```python
from build123d import *

# Parameters (mm, degrees)
LUMEN_REACH         = 11.007
SKETCH5_R           = 1.125
SKETCH6_R           = 3.044910248
SKETCH6_R_2         = 1.125
MINCHANNEL_DEPTH    = 6
BARBCHANNELFILLET_R = 1


with BuildPart() as part:
    # Sketch4 → Barb (revolve)
    with BuildSketch(Plane.XY, mode=Mode.PRIVATE) as barb_sk:
        Polygon((-8.593939394, 0), (-8.593939394, 4.75), (-2.593939394, 3.044910248), (-2.593939394, 0), align=None)
    revolve(barb_sk.sketch.rotate(Axis((0, 0, 0), (-1, 0, 0)), 90), axis=Axis((0, 0, 0), (-1, 0, 0)))

    # Sketch5 → Lumen (cut, up to next)
    with BuildSketch(Plane(origin=(-2.593939394, 0, 0), x_dir=(0, 0, -1), z_dir=(1, 0, 0)), mode=Mode.PRIVATE) as lumen_sk1:
        Circle(SKETCH5_R)
    lumen_tool1 = extrude(lumen_sk1.sketch, amount=-LUMEN_REACH, mode=Mode.PRIVATE) & part.part
    add(lumen_tool1.solids().sort_by_distance((-2.593939, 0, 0))[0], mode=Mode.SUBTRACT)

    # Sketch6 → MinChannel (add)
    with BuildSketch(Plane.ZY.offset(8.593939394)):
        Circle(SKETCH6_R)
        with Locations(Location((0, 0, 0), (0, 0, 180))):
            Circle(SKETCH6_R_2, mode=Mode.SUBTRACT)
    extrude(amount=MINCHANNEL_DEPTH)

    # BarbChannelFillet
    barbchannelfillet_edges = [part.edges().sort_by_distance(p)[0] for p in [
        (-8.593939394, 0, -3.044910248),
    ]]
    fillet(barbchannelfillet_edges, radius=BARBCHANNELFILLET_R)


solid = part.part
```
The listing builds one solid part. Answer for the finished solid, in the listing's coordinates (mm). A direction names the side the tool comes from. Coordinates: 2 decimals unless noted, no trailing zeros. Loops run counter-clockwise (first coordinate to the right, second up) from the corner with the lowest first, then second, coordinate; pieces in that order, holes last. Notation, with made-up numbers: M 47,29 L 69,29 A10 cw 69,33 Z; hole C 37,-2.75 d3. An arc over 180 degrees is marked long. Answer as a JSON object with one key per item and string values. Group by question number.
Item 1: Section C-C (x = -13) is taken. Write down the section's boundary in (y, z) (3 decimals), and give its area (3 significant figures).
Item 2: Consider L1, parallel to Y at x = -9.75, z = 0 (3 decimals); L2, parallel to Y at x = -9.25, z = 0 (3 decimals); L3, parallel to Z at x = -4.75, y = 1. Determine where each line is inside the solid, lowest interval first.
Item 3: Section A-A (y = 0) is taken. Write down the section's boundary in (x, z) (3 decimals), and give its area (3 significant figures).
Item 4: Determine the mould class of faces 3 (the face through (-8.51, -0.76, 0.83)), 4 (the face through (-12.059, 0.915, 2.904)), 5 (the face through (-14.594, -1.3, 0)) for opening direction Y: +Y half, -Y half, draft (parallel to the pull), parting line (faces both ways), or undercut.
Item 5: Which of the six approach directions +Z, -Z, +X, -X, +Y, -Y give full straight-line access (tool end or side, diameter ignored) to faces 1 (the face through (-2.594, 1.3, 0)), 2 (the face through (-8.594, -4, -2))?
Item 6: Section D-D (x = -6) is taken. Write down the section's boundary in (y, z) (3 decimals).
Item 7: Each of these flat-tipped pins is pushed along its axis until it touches: P1, Ø1, axis at y = 1, z = -3, coming from the +X side; P2, Ø1, axis at x = -5.5, y = -2, coming from the +Z side; P3, Ø4, axis at x = -6, z = -1.5, coming from the +Y side. Where does it stop, or does it pass through?
Solved:
{
 "1": {"outline": "C 0,0 d6.09; hole C 0,0 d2.25", "area": "25.2 mm2"},
 "2": {"L1": "y = -3.045 to -1.125, 1.125 to 3.045", "L2": "y = -3.106 to -1.125, 1.125 to 3.106", "L3": "z = -3.52 to -0.52, 0.52 to 3.52"},
 "3": {"outline": "M -14.594,-3.045 L -9.594,-3.045 A1 cw -8.594,-4.045 L -8.594,-4.75 L -2.594,-3.045 L -2.594,-1.125 L -14.594,-1.125 Z; M -14.594,1.125 L -2.594,1.125 L -2.594,3.045 L -8.594,4.75 L -8.594,4.045 A1 cw -9.594,3.045 L -14.594,3.045 Z", "area": "56.7 mm2"},
 "4": {"face 3": "undercut", "face 4": "parting line", "face 5": "draft"},
 "5": {"face 1": "+Z, -Z, +X, +Y, -Y", "face 2": "-X"},
 "6": {"outline": "C 0,0 d8.026; hole C 0,0 d2.25"},
 "7": {"P1": "stops at x = -2.59", "P2": "stops at z = 3.62", "P3": "stops at y = 4.48"}
}
